Design review of the part shown in the three views and the two pictorial views. Dimensions are in mm from the part's minimum x, y and z. A direction names the side the tool comes from. Coordinates: 2 decimals unless noted, no trailing zeros. Loops run counter-clockwise (first coordinate to the right, second up) from the corner with the lowest first, then second, coordinate; pieces in that order, holes last. Notation, with made-up numbers: M 69,12.5 L 108,12.5 A29 cw 108,46.5 Z; hole C -24.75,80 d11. An arc over 180 degrees is marked long. Write item = value, one per line. Start each with the question number.
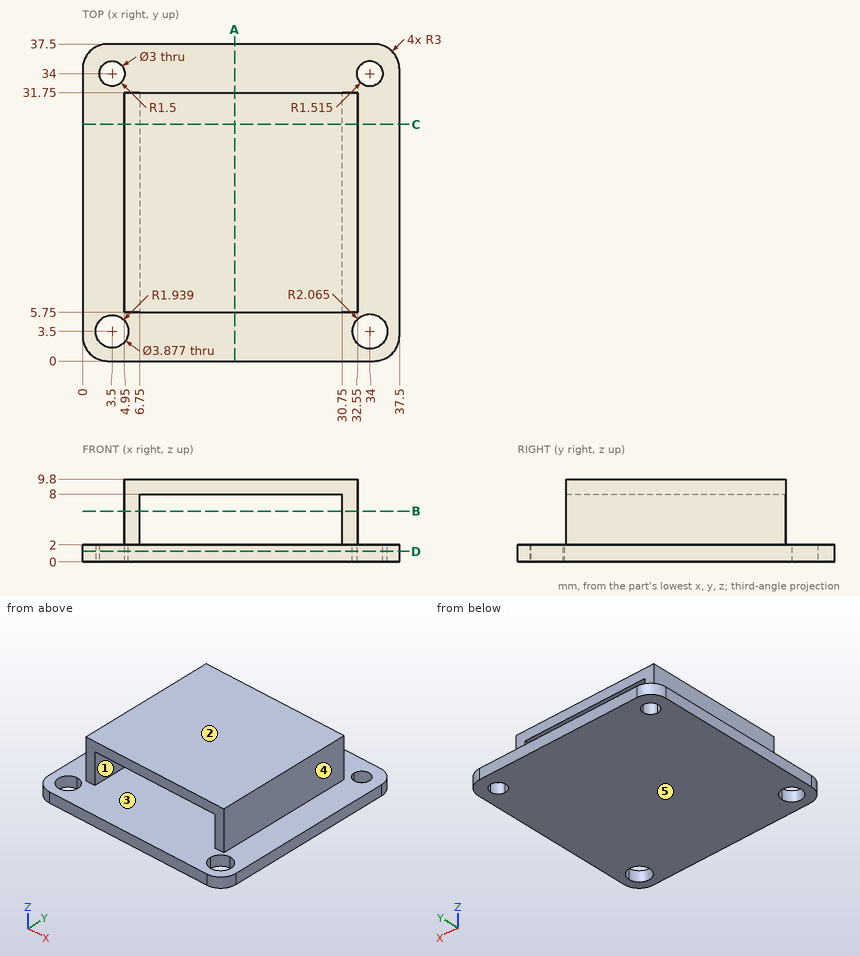
(1) Take a section at C-C (y = 28). State the section outline as (x, z) points.
(2) Take a section at A-A (x = 18). State the section outline as (y, z) points, plus the area to 3 significant figures.
(3) Insertion check: pin 1 (5 mm diameter, centred on x = 3.5, y = 34, fed in from +Z); pin 2 (2.5 mm diameter, centred on x = 21, z = 7, fed in from -Y); pin 3 (5 mm diameter, centred on y = 19.5, z = 6, fed in from -X). Each pin has a flat end and moves straight along its axis. Give the tip position at first contact, or say it passes through.
(4) Tool access review of the marked faces 1 and 2: name each direction out of +Z, -Z, +X, -X, +Y, -Y from which nothing blocks a thin tool from reaching the whole face with its end or side.
(5) To check wall thickness, follow L1, parallel to X at y = 34, z = 1.5 (1 decimal); L2, parallel to X at y = 3.5, z = 1.6 (1 decimal); L3, parallel to Y at x = 3.5, z = 0.6. State the ranges of each line that lie inside material, in increasing order.
(6) Take a section at D-D (z = 1.25). State the section outline as (x, y) points (1 decimal), plus the area to 3 significant figures.
(7) Take a section at B-B (z = 6). State the section outline as (x, y) points.
(8) Mouldability with a two-part tool opening along X and no side actions: class the marked faces 3, 4 and 5 as +X half, -X half, draft (parallel to the pull), parting line (faces both ways), or undercut.
Results list:
q1.outline = M 0,0 L 37.5,0 L 37.5,2 L 32.55,2 L 32.55,9.8 L 4.95,9.8 L 4.95,2 L 0,2 Z; hole M 6.75,2 L 30.75,2 L 30.75,8 L 6.75,8 Z
q2.outline = M 0,0 L 37.5,0 L 37.5,2 L 0,2 Z; M 5.75,8 L 31.75,8 L 31.75,9.8 L 5.75,9.8 Z
q2.area = 122 mm^2
q3.pin_1 = 2
q3.pin_2 = 5.75
q3.pin_3 = 4.95
q4.face_1 = +Y, -Y
q4.face_2 = +Z, +X, -X, +Y, -Y
q5.L1 = 0 to 2, 5 to 32.5, 35.5 to 37.5
q5.L2 = 0 to 1.6, 5.4 to 31.9, 36.1 to 37.5
q5.L3 = 0 to 1.56, 5.44 to 32.5, 35.5 to 37.5
q6.outline = M 0,3 A3 ccw 3,0 L 34.5,0 A3 ccw 37.5,3 L 37.5,34.5 A3 ccw 34.5,37.5 L 3,37.5 A3 ccw 0,34.5 Z; hole C 3.5,3.5 d3.9; hole C 3.5,34 d3; hole C 34,3.5 d4.1; hole C 34,34 d3
q6.area = 1,360 mm^2
q7.outline = M 4.95,5.75 L 6.75,5.75 L 6.75,31.75 L 4.95,31.75 Z; M 30.75,5.75 L 32.55,5.75 L 32.55,31.75 L 30.75,31.75 Z
q8.face_3 = undercut
q8.face_4 = +X half
q8.face_5 = draft
